Input: part model. Units: mm. Frame: model coordinates. Face numbers are marked on the shaded views. A direction names the side the tool comes from. Give positions to 0.01 mm unless a question says otherwise; leave off trailing zeros. Order: outer loops, then holes, each group sorted by start corner. A loop starts at its lowest first (then second) coordinate and runs counter-clockwise, first axis right, second up. Notation, with made-up numbers: (-32.75, 30) - (-18.75, 30) arc R11 ccw to (-18.75, 41) - close; hole circle Ø4 at (9, 79). An arc over 180 degrees is marked (long way). Answer in a Markdown table with one row per item. Add a question column.
1. Section query A-A on y = 9.5. Return loops of the section in (x, z), and give its area (3 significant figures).
2. Ray query, line 1 (Z direction, x = 12.7, y = 2.15); line 2 (Z direction, x = -6, y = 11.5). Return the intervals inside material, ascending. Write a range as [from, to].
3. Access query for the marked faces 1, 2 and 3. Directions: +Z, -Z, +X, -X, +Y, -Y. A direction counts if a zero-diameter tool reaches every point of the face in a straight line with its end or side. Return the directions, or none.
4. Section query D-D on x = 0. Return loops of the section in (y, z).
5. Section query C-C on x = -12.7. Return loops of the section in (y, z).
6. Contact query for flat-ended pins moving along their axis: pin 1 (5 mm diameter, centred on y = 8.5, z = 8, fed in from +X); pin 2 (4.5 mm diameter, centred on x = 2.5, y = 9, fed in from +Z); pin 3 (6 mm diameter, centred on x = -12.7, z = -12.7, fed in from +Y). Output: stop coordinate, or through.
7. Section query B-B on z = 0. Return loops of the section in (x, y), and give its area (3 significant figures).
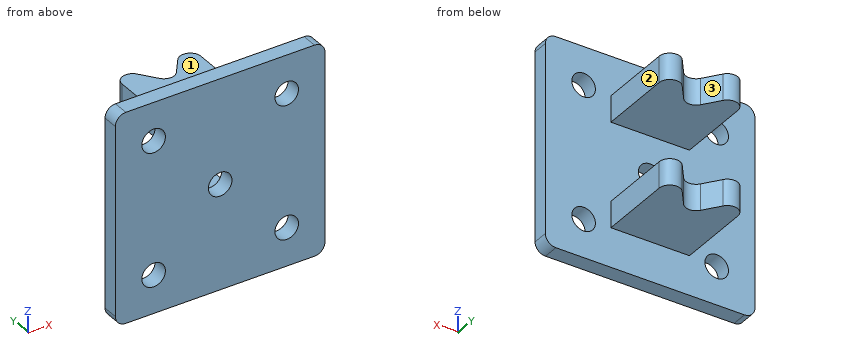
Autodesk Inventor part; units mm, degrees
ref_plane "YZ Plane" through (0, 0, 0) normal (1, 0, 0) x (0, 1, 0)
ref_plane "XZ Plane" through (0, 0, 0) normal (0, 1, 0) x (-1, 0, 0)
ref_plane "XY Plane" through (0, 0, 0) normal (0, 0, 1) x (1, 0, 0)
sketch "Sketch1" plane through (0, 0, 0) normal (0, 1, 0) x (-1, 0, 0)
  line L0 (-20, 20) -> (20, 20)
  line L1 (20, 20) -> (20, -20)
  line L2 (20, -20) -> (-20, -20)
  line L3 (-20, -20) -> (-20, 20)
  line L4 (-20, 20) -> (20, -20) construction
  line L5 (20, 20) -> (-20, -20) construction
  point P0 (0, 0)
  dimension "d0" = 40
  dimension "d1" = 40
extrude "Extrusion1" add sketch "Sketch1" along normal blind 3
sketch "Sketch2" plane through (0, 3, 0) normal (0, 1, 0) x (1, 0, 0)
  line L0 (-7.5, 12.5) -> (7.5, 12.5)
  line L1 (7.5, 12.5) -> (7.5, 7.5)
  line L2 (7.5, 7.5) -> (-7.5, 7.5)
  line L3 (-7.5, 7.5) -> (-7.5, 12.5)
  line L4 (-7.5, -7.5) -> (7.5, -7.5)
  line L5 (7.5, -7.5) -> (7.5, -12.5)
  line L6 (7.5, -12.5) -> (-7.5, -12.5)
  line L7 (-7.5, -12.5) -> (-7.5, -7.5)
  line L8 (0, 7.5) -> (0, -7.5) construction
  point P0 (-20, 20)
  point P1 (20, 20)
  point P2 (0, 0)
  point P3 (0, 0)
  dimension "d10" = 15
  dimension "d11" = 15
  dimension "d12" = 5
extrude "Extrusion2" add sketch "Sketch2" along normal blind 20
sketch "Sketch3" plane through (20, 0, -20) normal (0, 0, -1) x (-1, 0, 0)
  line L0 (40, 0) -> (0, 0)
  line L1 (12.5, 23) -> (27.5, 23)
  line L2 (12.5, 3) -> (12.5, 23)
  line L3 (12.5, 23) -> (20, 13)
  line L4 (20, 13) -> (27.5, 23)
  point P0 (20, 0)
  point P1 (20, 0)
  point P2 (20, 0)
  dimension "d13" = 10
extrude "Extrusion3" cut sketch "Sketch3" against normal through all
fillet "Fillet1" radius 2 10 edges at (0, 13, 10) (0, 13, -10) (-7.5, 23, -10) (-7.5, 23, 10) (7.5, 23, 10) (7.5, 23, -10) (20, 1.5, 20) (20, 1.5, -20) (-20, 1.5, -20) (-20, 1.5, 20)
sketch "Sketch5" plane through (0, 0, 0) normal (0, -1, 0) x (1, 0, 0)
  line L0 (12.7, -12.7) -> (-12.7, -12.7) construction
  line L1 (-12.7, -12.7) -> (-12.7, 12.7) construction
  point P0 (0, 0)
  point P1 (12.7, 12.7)
  point P2 (0, -12.7)
  point P3 (-12.7, 0)
  point P4 (0, 0)
  dimension "d14" = 25.4
  dimension "d15" = 25.4
hole "Hole1" at (12.7, 0, -12.7) at (-12.7, 0, -12.7) at (12.7, 0, 12.7) at (-12.7, 0, 12.7) at (0, 0, 0) direction (0, 1, 0) diameter 4.496 end through all
properties part number "CapillaryHolder"
Answer:
| question | item | result |
|---|---|---|
| 1 | outline | (-7.5, -12.5) - (7.5, -12.5) - (7.5, -7.5) - (-7.5, -7.5) - close; (-7.5, 7.5) - (7.5, 7.5) - (7.5, 12.5) - (-7.5, 12.5) - close |
| 1 | area | 150 mm² |
| 2 | line 1 | z = [-20, -14.95], [-10.45, 10.45], [14.95, 20] |
| 2 | line 2 | z = [-12.5, -7.5], [7.5, 12.5] |
| 3 | face 1 | +Z, +X, -X, +Y |
| 3 | face 2 | +Z, -Z, +X, +Y |
| 3 | face 3 | +Z, -Z, +Y |
| 4 | outline | (0, -20) - (3, -20) - (3, -12.5) - (14.33, -12.5) - (14.33, -7.5) - (3, -7.5) - (3, -2.25) - (0, -2.25) - close; (0, 2.25) - (3, 2.25) - (3, 7.5) - (14.33, 7.5) - (14.33, 12.5) - (3, 12.5) - (3, 20) - (0, 20) - close |
| 5 | outline | (0, -20) - (3, -20) - (3, -14.95) - (0, -14.95) - close; (0, -10.45) - (3, -10.45) - (3, 10.45) - (0, 10.45) - close; (0, 14.95) - (3, 14.95) - (3, 20) - (0, 20) - close |
| 6 | pin 1 | stops at x = 7.5 |
| 6 | pin 2 | stops at z = 12.5 |
| 6 | pin 3 | stops at y = 3 |
| 7 | outline | (-20, 0) - (-2.25, 0) - (-2.25, 3) - (-20, 3) - close; (2.25, 0) - (20, 0) - (20, 3) - (2.25, 3) - close |
| 7 | area | 107 mm² |
